```python
from build123d import *

# Parameters (mm, degrees)
SKETCH2_W               = 3
SKETCH2_H               = 9
CUT_EXTRUDE1_DEPTH      = 19.5
CUT_EXTRUDE1_DEPTH_BACK = 19.5
CHAMFER1_SIZE           = 1


with BuildPart() as part:
    # Sketch1 → Revolve1 (revolve)
    with BuildSketch(Plane.XY):
        Polygon((10.15, 100), (10.15, 33), (18.5, 33), (18.5, 23), (10.15, 23), (10.15, 0), (6.75, 0), (6.75, 100), align=None)
    revolve(axis=Axis((0, -728.004511314, 0), (0, 1, 0)))

    # Sketch2 → Cut-Extrude1 (cut, two sides)
    with BuildSketch(Plane.XY) as cut_extrude1_sk:
        with Locations((10.5, 10.5)):
            Rectangle(SKETCH2_W, SKETCH2_H)
        with Locations((-10.5, 10.5)):
            Rectangle(SKETCH2_W, SKETCH2_H)
    extrude(amount=CUT_EXTRUDE1_DEPTH, mode=Mode.SUBTRACT)
    extrude(cut_extrude1_sk.sketch, amount=-CUT_EXTRUDE1_DEPTH_BACK, mode=Mode.SUBTRACT)

    # Chamfer1
    chamfer1_edges = [part.edges().sort_by_distance(p)[0] for p in [
        (-18.5, 23, 0),
        (-18.5, 33, 0),
    ]]
    chamfer(chamfer1_edges, length=CHAMFER1_SIZE)


solid = part.part
```
Geometry: final body of the model. Coordinates: model frame, mm. A direction names the side the tool comes from. Coordinates: 2 decimals unless noted, no trailing zeros. Order: outer loops, then holes, each group sorted by start corner. A loop starts at its lowest first (then second) coordinate and runs counter-clockwise, first axis right, second up. Notation, with made-up numbers: (88.25, 79.5) -> (109.25, 79.5) arc R36 ccw to (109.25, 114.5) -> close; hole circle Ø1 at (24, -5.75). An arc over 180 degrees is marked (long way). Write item = value, one per line.
(1) Pull-direction query (X, two-part tool) for faces 1 (the flat face through (-8, 33, 8)), 2 (the cylindrical face through (-1.46, 50.7, 6.59)), 3 (the cylindrical face through (-8.05, 66.03, 6.18)); classes: pulls with the +X half, pulls with the -X half, needs draft (parallel to the pull), parting line crosses it, or undercut.
Solved:
face_1 = needs draft
face_2 = undercut
face_3 = parting line crosses it
(2) Cut plane B-B on x = 0. Return loops of the section in (y, z), plus the area to 3 significant figures.
Solved:
outline = (0, -10.15) -> (23, -10.15) -> (23, -17.5) -> (24, -18.5) -> (32, -18.5) -> (33, -17.5) -> (33, -10.15) -> (100, -10.15) -> (100, -6.75) -> (0, -6.75) -> close; (0, 6.75) -> (100, 6.75) -> (100, 10.15) -> (33, 10.15) -> (33, 17.5) -> (32, 18.5) -> (24, 18.5) -> (23, 17.5) -> (23, 10.15) -> (0, 10.15) -> close
area = 845 mm²
(3) Line query: line 1 (Z direction, x = 0, y = 55); line 2 (X direction, y = 94, z = 9). Output: solid intervals per line, ascending.
Solved:
line_1 = -10.15 to -6.75, 6.75 to 10.15
line_2 = -4.69 to 4.69
(4) Cut plane C-C on y = 87.5. Return loops of the section in (x, z).
Solved:
outline = circle Ø20.3 at (0, 0); hole circle Ø13.5 at (0, 0)
(5) Cut plane A-A on z = 0. Return loops of the section in (x, y).
Solved:
outline = (-18.5, 24) -> (-17.5, 23) -> (-10.15, 23) -> (-10.15, 15) -> (-9, 15) -> (-9, 6) -> (-10.15, 6) -> (-10.15, 0) -> (-6.75, 0) -> (-6.75, 100) -> (-10.15, 100) -> (-10.15, 33) -> (-17.5, 33) -> (-18.5, 32) -> close; (6.75, 0) -> (10.15, 0) -> (10.15, 6) -> (9, 6) -> (9, 15) -> (10.15, 15) -> (10.15, 23) -> (17.5, 23) -> (18.5, 24) -> (18.5, 32) -> (17.5, 33) -> (10.15, 33) -> (10.15, 100) -> (6.75, 100) -> close
(6) Pin query (flat end, axial travel): pin 1 Ø5 at (y, z) = (45.5, -11) entering from -X; pin 2 Ø10 at (x, y) = (3.5, 23) entering from -Z; pin 3 Ø2 at (x, y) = (3, 71.5) entering from +Z; pin 4 Ø8 at (x, z) = (0, 0) entering from +Y. Return the tip coordinate at first contact, or that it passes through.
Solved:
pin_1 = -5.55
pin_2 = -18.5
pin_3 = 9.95
pin_4 = through
(7) Access query for faces 4 (the flat face through (8, 23, 8)), 5 (the flat face through (9, 10, 0)), 6 (the flat face through (2, 0, 7)), 7 (the flat face through (-9, 10, 0)), 8 (the cylindrical face through (-4.01, 27.94, 18.06)). Directions: +Z, -Z, +X, -X, +Y, -Y. A direction counts if a zero-diameter tool reaches every point of the face in a straight line with its end or side. Return the directions, or none.
Solved:
face_4 = -Y
face_5 = +Z, -Z, +X
face_6 = +Z, -Z, +X, -X, -Y
face_7 = +Z, -Z, -X
face_8 = +Y, -Y
